```python
from build123d import *

# Parameters (mm, degrees)
SK_BODY_R          = 52
BODY_DRAFT1_DEPTH  = 56
BODY_DRAFT1_TAPER  = 1
SK_B20_R           = 10
CUT_B20_DEPTH      = 10
SK_PL0_W           = 27
SK_PL0_H           = 6.25
SK_CAV2_R          = 22
CUT_CAV44B_DEPTH   = 46
CUT_NOTCH120_DEPTH = 2
SK_H120_R          = 6.25
CUT_PL120C_DEPTH   = 26.9
CUT_NOTCH240_DEPTH = 2
SK_H240_R          = 6.25
CUT_PL240C_DEPTH   = 26.9
SK_P5_R            = 2.5
CUT_P5X3_DEPTH     = 22
CHAMFER_C1_SIZE    = 1
CHAMFER_C1_SIZE_2  = 0.982994102
CHAMFER_C1_SIZE_3  = 1.017920191
SK_M5V12_R         = 2.1
CUT_M5V12_DEPTH    = 16
SK_NOTCH90_W       = 2
SK_NOTCH90_H       = 0.8
CUT_NOTCH90_DEPTH  = 2
SK_OIL90_R         = 6.25
CUT_OIL90_DEPTH    = 22
SK_NOTCH270_W      = 2
SK_NOTCH270_H      = 0.8
CUT_NOTCH270_DEPTH = 2
CUT_OIL270_START   = 22
SK_OIL270_R        = 6.25
CUT_OIL270_DEPTH   = 22


with BuildPart() as part:
    # Sk_body → Body_draft1 (new body)
    with BuildSketch(Plane.XY):
        Circle(SK_BODY_R)
    extrude(amount=BODY_DRAFT1_DEPTH, taper=BODY_DRAFT1_TAPER)

    # Sk_b20 → Cut_b20 (cut)
    with BuildSketch(Plane.XY):
        Circle(SK_B20_R)
    extrude(amount=CUT_B20_DEPTH, mode=Mode.SUBTRACT)

    # Sk_pl0 → Cut_pl0 (revolve, cut)
    with BuildSketch(Plane.XY.offset(22), mode=Mode.PRIVATE) as cut_pl0_sk:
        with Locations((34.5, 3.125)):
            Rectangle(SK_PL0_W, SK_PL0_H)
    revolve(cut_pl0_sk.sketch.rotate(Axis((0, 0, 22), (1, 0, 0)), 90), axis=Axis((0, 0, 22), (1, 0, 0)), mode=Mode.SUBTRACT)

    # Sk_cav2 → Cut_cav44b (cut)
    with BuildSketch(Plane.XY.offset(10)):
        Circle(SK_CAV2_R)
    extrude(amount=CUT_CAV44B_DEPTH, mode=Mode.SUBTRACT)

    # Sk_notch120 → Cut_notch120 (cut)
    with BuildSketch(Plane.XY.offset(21)):
        Polygon((-24.466, 40.3764), (-22.734, 41.3764), (-23.134, 42.0692), (-24.866, 41.0692), align=None)
    extrude(amount=CUT_NOTCH120_DEPTH, mode=Mode.SUBTRACT)

    # Sk_h120 → Cut_pl120c (cut)
    with BuildSketch(Plane(origin=(-24.000519623, 41.568899987, 0), x_dir=(0.8660190526287386, 0.5000110003630143, 0), z_dir=(0.5000110003630142, -0.8660190526287385, 0))):
        with Locations(Location((0.000600013, 22, 0), (0, 0, 175.281583596))):
            Circle(SK_H120_R)
    extrude(amount=CUT_PL120C_DEPTH, mode=Mode.SUBTRACT)

    # Sk_notch240 → Cut_notch240 (cut)
    with BuildSketch(Plane.XY.offset(21)):
        Polygon((-22.734, -41.3764), (-24.466, -40.3764), (-24.866, -41.0692), (-23.134, -42.0692), align=None)
    extrude(amount=CUT_NOTCH240_DEPTH, mode=Mode.SUBTRACT)

    # Sk_h240 → Cut_pl240c (cut)
    with BuildSketch(Plane(origin=(-24.000519623, -41.568899987, 0), x_dir=(0.8660190526287386, -0.5000110003630143, 0), z_dir=(0.5000110003630142, 0.8660190526287385, 0))):
        with Locations(Location((0.000600013, -22, 0), (0, 0, 355.149686071))):
            Circle(SK_H240_R)
    extrude(amount=CUT_PL240C_DEPTH, mode=Mode.SUBTRACT)

    # Sk_p5 → Cut_p5x3 (cut)
    with BuildSketch(Plane.XY):
        with Locations(Location((26, 0, 0), (0, 0, 180))):
            Circle(SK_P5_R)
        with Locations(Location((-13, 22.5167, 0), (0, 0, 180))):
            Circle(SK_P5_R)
        with Locations(Location((-13, -22.5167, 0), (0, 0, 180))):
            Circle(SK_P5_R)
    extrude(amount=CUT_P5X3_DEPTH, mode=Mode.SUBTRACT)

    # Chamfer_C1
    # the kernel refuses this chamfer: 1.017920191, 1, 0.982994102 mm, written as the material it takes off along each edge
    with BuildSketch(Plane(origin=(0, 0, 56), x_dir=(1, 0, 0), z_dir=(0, -1, 0))) as chamfer_c1_piece_1:
        Polygon((22 + CHAMFER_C1_SIZE, 0), (22, -CHAMFER_C1_SIZE), (22, 0), align=None)
    revolve(axis=Axis((0, 0, 56), (0, 0, 1)), mode=Mode.SUBTRACT)
    with BuildSketch(Plane(origin=(0, 0, 10), x_dir=(1, 0, 0), z_dir=(0, -1, 0))) as chamfer_c1_piece_2:
        Polygon((10, -CHAMFER_C1_SIZE), (10 + CHAMFER_C1_SIZE, 0), (10, 0), align=None)
    revolve(axis=Axis((0, 0, 10), (0, 0, 1)), mode=Mode.SUBTRACT)
    with BuildSketch(Plane(origin=(0, 0, 0), x_dir=(1, 0, 0), z_dir=(0, -1, 0))) as chamfer_c1_piece_3:
        Polygon((10 + CHAMFER_C1_SIZE, 0), (10, CHAMFER_C1_SIZE), (10, 0), align=None)
    revolve(axis=Axis((0, 0, 0), (0, 0, 1)), mode=Mode.SUBTRACT)
    with BuildSketch(Plane(origin=(0, 0, 0), x_dir=(1, 0, 0), z_dir=(0, 1, 0))) as chamfer_c1_piece_4:
        Polygon((52 - CHAMFER_C1_SIZE, 0), (52 - CHAMFER_C1_SIZE_2 * 0.0174524064402, -CHAMFER_C1_SIZE_2 * 0.999847695326), (52, 0), align=None)
    revolve(axis=Axis((0, 0, 0), (0, 0, -1)), mode=Mode.SUBTRACT)
    with BuildSketch(Plane(origin=(0, 0, 56), x_dir=(1, 0, 0), z_dir=(0, 1, 0))) as chamfer_c1_piece_5:
        Polygon((51.022516364 + CHAMFER_C1_SIZE * 0.0174524064373, CHAMFER_C1_SIZE * 0.999847695156), (51.022516364 - CHAMFER_C1_SIZE_3, 0), (51.022516364, 0), align=None)
    revolve(axis=Axis((0, 0, 56), (0, 0, -1)), mode=Mode.SUBTRACT)

    # Sk_m5v12 → Cut_m5v12 (cut)
    with BuildSketch(Plane.XY.offset(40)):
        with Locations((44, 0)):
            Circle(SK_M5V12_R)
        with Locations((22, 38.1051)):
            Circle(SK_M5V12_R)
        with Locations((-22, 38.1051)):
            Circle(SK_M5V12_R)
        with Locations((-44, 0)):
            Circle(SK_M5V12_R)
        with Locations((-22, -38.1051)):
            Circle(SK_M5V12_R)
        with Locations((22, -38.1051)):
            Circle(SK_M5V12_R)
    extrude(amount=CUT_M5V12_DEPTH, mode=Mode.SUBTRACT)

    # Sk_notch90 → Cut_notch90 (cut)
    with BuildSketch(Plane.XY.offset(39)):
        with Locations((0, 30.4)):
            Rectangle(SK_NOTCH90_W, SK_NOTCH90_H)
    extrude(amount=CUT_NOTCH90_DEPTH, mode=Mode.SUBTRACT)

    # Sk_oil90 → Cut_oil90 (cut)
    with BuildSketch(Plane(origin=(0, 30, 0), x_dir=(1, 0, 0), z_dir=(0, 1, 0))):
        with Locations(Location((0, -40, 0), (0, 0, 135.962349207))):
            Circle(SK_OIL90_R)
    extrude(amount=CUT_OIL90_DEPTH, mode=Mode.SUBTRACT)

    # Sk_notch270 → Cut_notch270 (cut)
    with BuildSketch(Plane.XY.offset(39)):
        with Locations((0, -30.4)):
            Rectangle(SK_NOTCH270_W, SK_NOTCH270_H)
    extrude(amount=CUT_NOTCH270_DEPTH, mode=Mode.SUBTRACT)

    # Sk_oil270 → Cut_oil270 (cut)
    with BuildSketch(Plane.XZ.offset(30).offset(CUT_OIL270_START)):
        with Locations(Location((0, 40, 0), (0, 0, 224.037650793))):
            Circle(SK_OIL270_R)
    extrude(amount=-CUT_OIL270_DEPTH, mode=Mode.SUBTRACT)


solid = part.part
```
Check sheet for the modelled part. Datum: model origin and axes. Units: mm. A direction names the side the tool comes from. Coordinates: 2 decimals unless noted, no trailing zeros. Order: outer loops, then holes, each group sorted by start corner. A loop starts at its lowest first (then second) coordinate and runs counter-clockwise, first axis right, second up. Notation, with made-up numbers: M 51,13 L 55,13 A16 cw 55,22 Z; hole C -10.5,3.5 d2. An arc over 180 degrees is marked long. One line per question, with ' | ' between items. Start each with the question number.
Item 1: Material ranges on line 1 (Y direction, x = -28.5, z = 25); line 2 (X direction, y = -1, z = 19.5); line 3 (Y direction, x = 44, z = 44), recorded low to high.
Item 2: Sectioned sample at D-D on z = 42. Record the cut outline in (x, y).
Item 3: Sectioned sample at B-B on z = 48.5. Record the cut outline in (x, y).
Item 4: Sectioned sample at A-A on z = 24.5. Record the cut outline in (x, y).
Item 5: Access from +Z, -Z, +X, -X, +Y, -Y to the whole of each face (thin tool, end or side, straight path). Record for faces 1 (the cylindrical face through (1.78, 40.56, 34.01)), 2 (the cylindrical face through (34.74, -1.88, 27.96)), 3 (the flat face through (-22, -38, 40)).
Item 6: Gauge pin test, flat ends, axial feed: P1, Ø8, axis at y = -34.5, z = 26.5, coming from the -X side; P2, Ø7.5, axis at y = 0, z = 22, coming from the +X side; P3, Ø10, axis at y = 18, z = 36.5, coming from the +X side. Record the tip position at first contact, or that the pin passes through.
Item 7: Mould release check, pull along Z, two halves, no side actions. Record for faces 4 (the flat face through (-1, 12, 0)), 5 (the flat face through (-22, 38, 40)), 6 (the cylindrical face through (28.5, -0.1, 8)), 7 (the cylindrical face through (0.92, -40.86, 46.18)): pulls with the +Z half, pulls with the -Z half, needs draft (parallel to the pull), parting line crosses it, or undercut.
Item 8: Sectioned sample at C-C on x = -13. Count the separate pieces of the cut face and the enclosed holes in it, and give its area (3 significant figures).
Answer below:
1) line 1: y = -42.97 to -38.97, -38.4 to 38.4, 38.97 to 42.97 | line 2: x = -51.65 to -21.98, 48 to 51.65 | line 3: y = -26.24 to -2.1, 2.1 to 26.24
2) outline: M -5.92,-50.92 L -5.92,-30 L 5.92,-30 L 5.92,-50.92 A51.27 ccw 5.92,50.92 L 5.92,30 L -5.92,30 L -5.92,50.92 A51.27 ccw Z; hole C -44,0 d4.2; hole C -22,-38.11 d4.2; hole C -22,38.11 d4.2; hole C 0,0 d44; hole C 22,-38.11 d4.2; hole C 22,38.11 d4.2; hole C 44,0 d4.2
3) outline: C 0,0 d102.31; hole C -44,0 d4.2; hole C -22,-38.11 d4.2; hole C -22,38.11 d4.2; hole C 0,0 d44; hole C 22,-38.11 d4.2; hole C 22,38.11 d4.2; hole C 44,0 d4.2
4) outline: C 0,0 d103.14; hole M -28.96,-38.71 L -19.04,-44.43 L -5.66,-21.26 A22 ccw 21.24,-5.73 L 48,-5.73 L 48,5.73 L 21.24,5.73 A22 ccw -5.66,21.26 L -19.04,44.43 L -28.96,38.71 L -15.58,15.53 A22 ccw -15.58,-15.53 Z
5) face 1: +Y | face 2: none | face 3: +Z
6) P1: stops at x = -41.54 | P2: stops at x = 51.68 | P3: stops at x = 49.69
7) face 4: pulls with the -Z half | face 5: pulls with the +Z half | face 6: needs draft | face 7: undercut
8) separate pieces: 3 | enclosed holes: 0 | area: 3,430 mm^2
